For this review, take the finished solid that the model builds, in its own axes (mm). A direction names the side the tool comes from. Coordinates: 2 decimals unless noted, no trailing zeros. Write each loop counter-clockwise with the first axis right and the second up, starting at its lowest first coordinate (ties: lowest second). Pieces come first, ordered by that corner, then holes.
```python
from build123d import *

# Parameters (mm, degrees)
EXTRUDE1_DEPTH = 54
EXTRUDE2_DEPTH = 47.019237886


with BuildPart() as part:
    # Sketch1 → Extrude1 (new body)
    with BuildSketch(Plane.XY):
        with BuildLine():
            Line((0, 0), (0, 70))
            Line((0, 70), (24.019237886, 70))
            ThreePointArc((24.019237886, 70), (39.575587073, 63.556349186), (46.019237886, 48))
            Line((46.019237886, 48), (46.019237886, 24))
            Line((46.019237886, 24), (72, 9))
            Line((72, 9), (72, 0))
            Line((72, 0), (0, 0))
        make_face()
    extrude(amount=EXTRUDE1_DEPTH)

    # Sketch2 → Extrude2 (cut, through all)
    with BuildSketch(Plane(origin=(46.019237886, 0, 0), x_dir=(0, 0, -1), z_dir=(1, 0, 0))):
        Polygon((-54, 24), (-22, 70), (-54, 70), align=None)
    extrude(amount=-EXTRUDE2_DEPTH, mode=Mode.SUBTRACT)


solid = part.part
```
Q1. Add section A-A (z = 7). State the section outline as (x, y) points, then the cut area to 3 significant figures.
Ans:
outline: (0, 0) - (72, 0) - (72, 9) - (46.02, 24) - (46.02, 48) arc R22 ccw to (24.02, 70) - (0, 70) - close
area: 3,550 mm2
Q2. For probe 1 along X at (y, z) = (35, 46); probe 2 along Y at (x, z) = (49.5, 18); probe 3 along X at (y, z) = (20, 12), list the stretches that pass through material, from the lowest coordinate up.
Ans:
probe 1: x = 0 to 46.02
probe 2: y = 0 to 21.99
probe 3: x = 0 to 52.95
Q3. Tool access review of faces 1 (the flat face through (37, 12, 54)), 2 (the flat face through (46.019, 36, 21)): name each direction out of +Z, -Z, +X, -X, +Y, -Y from which nothing blocks a thin tool from reaching the whole face with its end or side.
Ans:
face 1: +Z, +X, -X, +Y, -Y
face 2: +Z, -Z, +X, +Y
Q4. Clearance check with flat-ended pins moving along their axes: pin 1 Ø12 at (x, y) = (23, 38.5) entering from +Z; pin 2 Ø5 at (y, z) = (45, 5.5) entering from +X; pin 3 Ø5 at (x, y) = (40.5, 36.5) entering from +Z. State where each tip first meets the part, or that it passes through.
Ans:
pin 1: stops at z = 48.09
pin 2: stops at x = 46.02
pin 3: stops at z = 47.04
Q5. Add section D-D (x = 42.5). State the section outline as (y, z) points, then the cut area to 3 significant figures.
Ans:
outline: (0, 0) - (59.94, 0) - (59.94, 29) - (24, 54) - (0, 54) - close
area: 2,790 mm2
Q6. Add section B-B (x = 5). State the section outline as (y, z) points, then the cut area to 3 significant figures.
Ans:
outline: (0, 0) - (70, 0) - (70, 22) - (24, 54) - (0, 54) - close
area: 3,040 mm2
Q7. Add section C-C (y = 10). State the section outline as (x, z) points, then the cut area to 3 significant figures.
Ans:
outline: (0, 0) - (70.27, 0) - (70.27, 54) - (0, 54) - close
area: 3,790 mm2
